CAD build for the part. Positions are in the model's coordinates, mm. A direction names the side the tool comes from. Round coordinates to 2 decimals unless told otherwise and drop trailing zeros. Order: outer loops, then holes, each group sorted by start corner. A loop starts at its lowest first (then second) coordinate and runs counter-clockwise, first axis right, second up. Notation, with made-up numbers: M 24.5,0 L 45.5,0 A27 ccw 45.5,30 Z; hole C 86,-22.5 d9. An arc over 180 degrees is marked long. Put each result on its own line as item: value.
```python
from build123d import *

# Parameters (mm, degrees)
BOSS_EXTRUDE1_DEPTH = 66
CUT_EXTRUDE2_DEPTH  = 10
SKETCH3_R           = 3.5
CUT_EXTRUDE3_DEPTH  = 10
CHAMFER1_SIZE       = 0.5


with BuildPart() as part:
    # Sketch1 → Boss-Extrude1 (new body)
    with BuildSketch(Plane.XY):
        with BuildLine():
            Line((0, 29), (52, 29))
            ThreePointArc((52, 29), (56.242640687, 27.242640687), (58, 23))
            Line((58, 23), (58, 0))
            Line((58, 0), (62, 0))
            Line((62, 0), (62, 23))
            ThreePointArc((62, 23), (59.071067812, 30.071067812), (52, 33))
            Line((52, 33), (0, 33))
            Line((0, 33), (0, 29))
        make_face()
    extrude(amount=BOSS_EXTRUDE1_DEPTH)

    # Sketch2 → Cut-Extrude2 (cut)
    with BuildSketch(Plane(origin=(0, 33, 0), x_dir=(1, 0, 0), z_dir=(0, 1, 0))):
        with BuildLine():
            Line((28, -30), (31.803847577, -30))
            ThreePointArc((31.803847577, -30), (43, -33), (31.803847577, -36))
            Line((31.803847577, -36), (28, -36))
            ThreePointArc((28, -36), (25, -33), (28, -30))
        make_face()
    extrude(amount=-CUT_EXTRUDE2_DEPTH, mode=Mode.SUBTRACT)

    # Sketch3 → Cut-Extrude3 (cut)
    with BuildSketch(Plane(origin=(0, 33, 0), x_dir=(1, 0, 0), z_dir=(0, 1, 0))):
        with Locations(Location((10, -33, 0), (0, 0, 270))):
            Circle(SKETCH3_R)
    extrude(amount=-CUT_EXTRUDE3_DEPTH, mode=Mode.SUBTRACT)

    # Chamfer1
    chamfer1_edges = [part.edges().sort_by_distance(p)[0] for p in [
        (10, 33, 29.5),
    ]]
    chamfer(chamfer1_edges, length=CHAMFER1_SIZE)


solid = part.part
```
Item 1: Probe line 1 along Z through (x, y) = (37, 31); line 2 along X through (y, z) = (30, 33); line 3 along X through (y, z) = (30.1, 33). List the from-to ranges inside material, lowest first. Write a range as [from, to].
Answers below:
line 1: [0, 27], [39, 66]
line 2: [0, 6.5], [13.5, 25], [43, 59.14]
line 3: [0, 6.5], [13.5, 25], [43, 59.04]
Item 2: Band-saw the part on D-D on x = 37. Give the cut face in (y, z).
Answers below:
outline: M 29,0 L 33,0 L 33,27 L 29,27 Z; M 29,39 L 33,39 L 33,66 L 29,66 Z
Item 3: Pin check, flat tips, straight feed: P1, Ø18.5, axis at y = 8, z = 26, coming from the -X side; P2, Ø19, axis at x = 37, z = 33, coming from the +Y side; P3, Ø3, axis at y = 22.5, z = 36, coming from the -X side; P4, Ø4, axis at x = 51, z = 30, coming from the -Y side. Stop position of each tip, or through.
Answers below:
P1: x = 58
P2: y = 33
P3: x = 57.92
P4: y = 28.92
Item 4: Band-saw the part on C-C on z = 14. Give the cut face in (x, y).
Answers below:
outline: M 0,29 L 52,29 A6 cw 58,23 L 58,0 L 62,0 L 62,23 A10 ccw 52,33 L 0,33 Z
Item 5: Tool access for faces 5 (the cylindrical face through (59.15, 29.99, 32.54)), 6 (the flat face through (30, 31, 30)), 7 (the flat face through (58, 12, 33)): list every direction of +Z, -Z, +X, -X, +Y, -Y with a clear straight run to the whole face (end or side of a thin tool).
Answers below:
face 5: +Z, -Z, +X, +Y
face 6: +Y, -Y
face 7: +Z, -Z, -X, -Y
Item 6: Band-saw the part on B-B on x = 10. Give the cut face in (y, z), and give its area (3 significant figures).
Answers below:
outline: M 29,0 L 33,0 L 33,29 L 32.5,29.5 L 29,29.5 Z; M 29,36.5 L 32.5,36.5 L 33,37 L 33,66 L 29,66 Z
area: 236 mm²
Item 7: Band-saw the part on A-A on z = 33. Give the cut face in (x, y).
Answers below:
outline: M 0,29 L 6.5,29 L 6.5,32.5 L 6,33 L 0,33 Z; M 13.5,29 L 25,29 L 25,33 L 14,33 L 13.5,32.5 Z; M 43,29 L 52,29 A6 cw 58,23 L 58,0 L 62,0 L 62,23 A10 ccw 52,33 L 43,33 Z
Item 8: Mould opens along Z. For faces 1 (the flat face through (30, 31, 36)), 2 (the flat face through (40, 30, 66)), 3 (the flat face through (20, 29, 33)), 4 (the cylindrical face through (25, 31, 33)) say: pulls with the +Z half, pulls with the -Z half, needs draft (parallel to the pull), parting line crosses it, or undercut.
Answers below:
face 1: undercut
face 2: pulls with the +Z half
face 3: needs draft
face 4: undercut
